Build history of the part. All positions in model axes, mm. A direction names the side the tool comes from. Round coordinates to 2 decimals unless told otherwise and drop trailing zeros. Order: outer loops, then holes, each group sorted by start corner. A loop starts at its lowest first (then second) coordinate and runs counter-clockwise, first axis right, second up. Notation, with made-up numbers: M 15.5,45 L 67.5,45 A23 cw 67.5,59 Z; hole C 70.5,-3.75 d1. An arc over 180 degrees is marked long. Use CSV: the item, a comma, the result in double quotes.
from build123d import *

# Parameters (mm, degrees)
SKETCH1_W                                            = 190
SKETCH1_H                                            = 32
BOSS_EXTRUDE1_DEPTH                                  = 16
CHAMFER1_SIZE                                        = 2
SKETCH2_W                                            = 25
SKETCH2_H                                            = 4
CUT_EXTRUDE1_DEPTH                                   = 33
M12_TAPPED_HOLE1_D                                   = 10.2
M12_TAPPED_HOLE1_DEPTH                               = 24
M12_TAPPED_HOLE1_CSINK_D                             = 12.05
M12_TAPPED_HOLE1_CSINK_ANGLE                         = 90
M12_TAPPED_HOLE1_TIP                                 = 3.064389157
M4_TAPPED_HOLE1_D                                    = 3.3
M4_TAPPED_HOLE1_DEPTH                                = 11.5
M4_TAPPED_HOLE1_CSINK_D                              = 4.05
M4_TAPPED_HOLE1_CSINK_ANGLE                          = 90
M4_TAPPED_HOLE1_TIP                                  = 0.991420021
CSK_FOR_M10_COUNTERSUNK_FLAT_HEAD_SCREW1_D           = 6.5
CSK_FOR_M10_COUNTERSUNK_FLAT_HEAD_SCREW1_CSINK_D     = 13
CSK_FOR_M10_COUNTERSUNK_FLAT_HEAD_SCREW1_CSINK_ANGLE = 90
SKETCH12_R                                           = 3
CUT_EXTRUDE2_DEPTH                                   = 33
CSK_FOR_M4_COUNTERSUNK_FLAT_HEAD_SCREW1_D            = 1.5
CSK_FOR_M4_COUNTERSUNK_FLAT_HEAD_SCREW1_DEPTH        = 11.5
CSK_FOR_M4_COUNTERSUNK_FLAT_HEAD_SCREW1_CSINK_D      = 4
CSK_FOR_M4_COUNTERSUNK_FLAT_HEAD_SCREW1_CSINK_ANGLE  = 90
CSK_FOR_M4_COUNTERSUNK_FLAT_HEAD_SCREW1_TIP          = 0.450645464
M4_TAPPED_HOLE2_D                                    = 3.3
M4_TAPPED_HOLE2_DEPTH                                = 16
M4_TAPPED_HOLE2_TIP                                  = 0.991420021
SKETCH19_R                                           = 3
CUT_EXTRUDE3_DEPTH                                   = 33


with BuildPart() as part:
    # Sketch1 → Boss-Extrude1 (new body, symmetric)
    with BuildSketch(Plane.XY):
        Rectangle(SKETCH1_W, SKETCH1_H)
    extrude(amount=BOSS_EXTRUDE1_DEPTH, both=True)

    # Chamfer1
    chamfer1_edges = [part.edges().sort_by_distance(p)[0] for p in [
        (-95, 0, 16),
        (95, 0, 16),
        (-95, 0, -16),
    ]]
    chamfer(chamfer1_edges, length=CHAMFER1_SIZE)

    # Sketch2 → Cut-Extrude1 (cut, through all)
    with BuildSketch(Plane(origin=(0, 16, 0), x_dir=(1, 0, 0), z_dir=(0, 1, 0))):
        with Locations((79.5, 14)):
            Rectangle(SKETCH2_W, SKETCH2_H)
    extrude(amount=-CUT_EXTRUDE1_DEPTH, mode=Mode.SUBTRACT)

    # M12 Tapped Hole1
    with Locations(Plane(origin=(0, 16, 0), x_dir=(1, 0, 0), z_dir=(0, 1, 0))):
        with Locations((-63, 0), (11, 0)):
            CounterSinkHole(M12_TAPPED_HOLE1_D / 2, M12_TAPPED_HOLE1_CSINK_D / 2, depth=M12_TAPPED_HOLE1_DEPTH, counter_sink_angle=M12_TAPPED_HOLE1_CSINK_ANGLE)
            with Locations((0, 0, -(M12_TAPPED_HOLE1_DEPTH + M12_TAPPED_HOLE1_TIP / 2))):  # 118° drill point
                Cone(0, M12_TAPPED_HOLE1_D / 2, M12_TAPPED_HOLE1_TIP, mode=Mode.SUBTRACT)

    # M4 Tapped Hole1
    with Locations(Plane.XY.offset(16)):
        with Locations((-63, 4), (11, 4)):
            CounterSinkHole(M4_TAPPED_HOLE1_D / 2, M4_TAPPED_HOLE1_CSINK_D / 2, depth=M4_TAPPED_HOLE1_DEPTH, counter_sink_angle=M4_TAPPED_HOLE1_CSINK_ANGLE)
            with Locations((0, 0, -(M4_TAPPED_HOLE1_DEPTH + M4_TAPPED_HOLE1_TIP / 2))):  # 118° drill point
                Cone(0, M4_TAPPED_HOLE1_D / 2, M4_TAPPED_HOLE1_TIP, mode=Mode.SUBTRACT)

    # CSK for M10 Countersunk Flat Head Screw1 (through all)
    with Locations(Plane.XY.offset(16)):
        with Locations((77.5, 4)):
            CounterSinkHole(CSK_FOR_M10_COUNTERSUNK_FLAT_HEAD_SCREW1_D / 2, CSK_FOR_M10_COUNTERSUNK_FLAT_HEAD_SCREW1_CSINK_D / 2, counter_sink_angle=CSK_FOR_M10_COUNTERSUNK_FLAT_HEAD_SCREW1_CSINK_ANGLE)

    # Sketch12 → Cut-Extrude2 (cut, through all)
    with BuildSketch(Plane.XY.offset(16)):
        with Locations((-87, 6)):
            Circle(SKETCH12_R)
    extrude(amount=-CUT_EXTRUDE2_DEPTH, mode=Mode.SUBTRACT)

    # CSK for M4 Countersunk Flat Head Screw1
    with Locations(Plane(origin=(0, 16, 0), x_dir=(1, 0, 0), z_dir=(0, 1, 0))):
        with Locations((-87, 0)):
            CounterSinkHole(CSK_FOR_M4_COUNTERSUNK_FLAT_HEAD_SCREW1_D / 2, CSK_FOR_M4_COUNTERSUNK_FLAT_HEAD_SCREW1_CSINK_D / 2, depth=CSK_FOR_M4_COUNTERSUNK_FLAT_HEAD_SCREW1_DEPTH, counter_sink_angle=CSK_FOR_M4_COUNTERSUNK_FLAT_HEAD_SCREW1_CSINK_ANGLE)
            with Locations((0, 0, -(CSK_FOR_M4_COUNTERSUNK_FLAT_HEAD_SCREW1_DEPTH + CSK_FOR_M4_COUNTERSUNK_FLAT_HEAD_SCREW1_TIP / 2))):  # 118° drill point
                Cone(0, CSK_FOR_M4_COUNTERSUNK_FLAT_HEAD_SCREW1_D / 2, CSK_FOR_M4_COUNTERSUNK_FLAT_HEAD_SCREW1_TIP, mode=Mode.SUBTRACT)

    # M4 Tapped Hole2
    with Locations(Plane(origin=(0, 16, 0), x_dir=(1, 0, 0), z_dir=(0, 1, 0))):
        with Locations((-43, 0)):
            Hole(M4_TAPPED_HOLE2_D / 2, depth=M4_TAPPED_HOLE2_DEPTH)
            with Locations((0, 0, -(M4_TAPPED_HOLE2_DEPTH + M4_TAPPED_HOLE2_TIP / 2))):  # 118° drill point
                Cone(0, M4_TAPPED_HOLE2_D / 2, M4_TAPPED_HOLE2_TIP, mode=Mode.SUBTRACT)

    # Sketch19 → Cut-Extrude3 (cut, through all)
    with BuildSketch(Plane(origin=(0, 16, 0), x_dir=(1, 0, 0), z_dir=(0, 1, 0))):
        with Locations((-37, 10)):
            Circle(SKETCH19_R)
        with Locations((37, 10)):
            Circle(SKETCH19_R)
    extrude(amount=-CUT_EXTRUDE3_DEPTH, mode=Mode.SUBTRACT)


solid = part.part
(1) Cut at A-A, the plane x = 77.5. Give the cut face in (y, z).
Answer block:
outline,"M -16,-12 L 0.75,-12 L 0.75,12.75 L -2.5,16 L -16,16 Z; M 7.25,-12 L 16,-12 L 16,16 L 10.5,16 L 7.25,12.75 Z"
(2) Cut at B-B, the plane y = -13.5. Give the cut face in (x, z), and give its area (3 significant figures).
Answer block:
outline,"M -95,-14 L -93,-16 L 67,-16 L 67,-12 L 92,-12 L 92,-16 L 95,-16 L 95,14 L 93,16 L -93,16 L -95,14 Z; hole C -37,-10 d6; hole C 37,-10 d6"
area,"5,920 mm²"
(3) Wall check: line 1 (X direction, y = -2, z = -10); line 2 (X direction, y = -5, z = -4); line 3 (Z direction, x = -37, y = 1). Give the ranges that are in metal, low to high. Write a range as from..to.
Answer block:
line 1,"x = -95..-40, -34..34, 40..95"
line 2,"x = -95..-66.16, -59.84..7.84, 14.16..95"
line 3,"z = -16..-13, -7..16"
(4) Tool access for faces 1 (the face through (9.476, 3.368, 10.146)), 2 (the face through (92, 0, -14)), 3 (the face through (8.26, 3.38, -4.3)): list every direction of +Z, -Z, +X, -X, +Y, -Y with a clear straight run to the whole face (end or side of a thin tool).
Answer block:
face 1,"+Z"
face 2,"-Z, +Y, -Y"
face 3,"+Y"
(5) Cut at C-C, the plane y = -5.5. Give the cut face in (x, z).
Answer block:
outline,"M -95,-14 L -93,-16 L 67,-16 L 67,-12 L 92,-12 L 92,-16 L 95,-16 L 95,14 L 93,16 L -93,16 L -95,14 Z; hole C -63,0 d10.2; hole C -37,-10 d6; hole C 11,0 d10.2; hole C 37,-10 d6"
(6) Cut at D-D, the plane x = -37. Give the cut face in (y, z).
Answer block:
outline,"M -16,-16 L 16,-16 L 16,-13 L -16,-13 Z; M -16,-7 L 16,-7 L 16,16 L -16,16 Z"
(7) Drop flat-ended pins along their axis: pin 1 (7.5 mm diameter, centred on x = 74, y = 5.5, fed in from -Z); pin 2 (0.9 mm diameter, centred on x = -87, z = 0, fed in from +Y). Give the stop position or say it passes through.
Answer block:
pin 1,"stops at z = -12"
pin 2,"stops at y = 3.03"
(8) Two-plate mould, pull along Y, no slides. Class faces 4 (the face through (-61.35, 4.07, 10.15)), 5 (the face through (93, 0, -16)), 6 (the face through (-43.286, -0.819, -0.013)): released by +Y, released by -Y, zero draft, split by the parting line, or undercut.
Answer block:
face 4,"undercut"
face 5,"zero draft"
face 6,"released by +Y"
